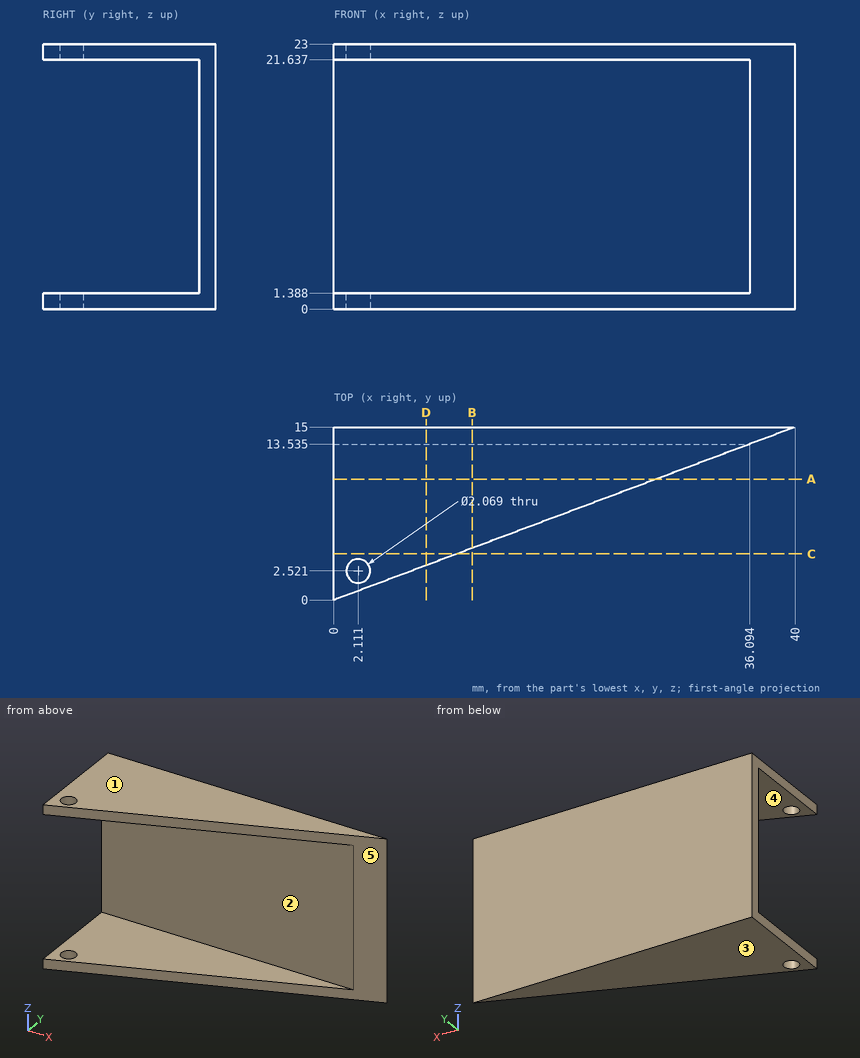
Input: dimensioned drawing with shaded views. Units: mm. Origin: part minimum x, y, z. A direction names the side the tool comes from. Give positions to 0.01 mm unless a question says otherwise; leave off trailing zeros. Write each loop counter-clockwise with the first axis right and the second up, starting at its lowest first coordinate (ties: lowest second). Pieces come first, ordered by that corner, then holes.
Q1. Section D-D, the plane x = 8. Output: boundary loops of the cut face in (y, z) (1 decimal).
Q2. Section B-B, the plane x = 12. Output: boundary loops of the cut face in (y, z) (1 decimal).
Q3. Pull-direction query (Z, two-part tool) for the marked faces 1, 2 and 3; classes: pulls with the +Z half, pulls with the -Z half, needs draft (parallel to the pull), parting line crosses it, or undercut.
Q4. Section C-C, the plane y = 4. Output: boundary loops of the cut face in (x, z).
Q5. First-contact query: P1, Ø7, axis at x = 15, y = 10, coming from the -Z side; P2, Ø10, axis at x = 17, z = 8.5, coming from the -Y side (1 decimal). Flat tips, straight axial feed; report the tip coordinate or a pass-through.
Q6. Material intervals for probe 1 along Z at (x, y) = (21, 8); probe 2 along Y at (x, z) = (16, 21) (1 decimal); probe 3 along Y at (x, z) = (27, 22.25) (1 decimal), sorted ascending.
Q7. Set-up query: the marked faces 4 and 5. Return all of +Z, -Z, +X, -X, +Y, -Y with unobstructed straight access to the full face (end or side cutting, diameter ignored); none if empty.
Q8. Section A-A, the plane y = 10.5. Output: boundary loops of the cut face in (x, z).
Filled in:
1. outline: (3, 0) - (15, 0) - (15, 23) - (3, 23) - (3, 21.6) - (13.5, 21.6) - (13.5, 1.4) - (3, 1.4) - close
2. outline: (4.5, 0) - (15, 0) - (15, 23) - (4.5, 23) - (4.5, 21.6) - (13.5, 21.6) - (13.5, 1.4) - (4.5, 1.4) - close
3. face 1: pulls with the +Z half
3. face 2: undercut
3. face 3: pulls with the -Z half
4. outline: (0, 0) - (10.67, 0) - (10.67, 1.39) - (0, 1.39) - close; (0, 21.64) - (10.67, 21.64) - (10.67, 23) - (0, 23) - close
5. P1: stops at z = 0
5. P2: stops at y = 13.5
6. probe 1: z = 0 to 1.39, 21.64 to 23
6. probe 2: y = 13.5 to 15
6. probe 3: y = 10.1 to 15
7. face 4: +X, -X, -Y
7. face 5: +Z, -Z, +X, -Y
8. outline: (0, 0) - (28, 0) - (28, 1.39) - (0, 1.39) - close; (0, 21.64) - (28, 21.64) - (28, 23) - (0, 23) - close
